from build123d import *

# Parameters (mm, degrees)
SKETCH_1_W          = 20
SKETCH_1_H          = 145
EXTRUDE_1_DEPTH     = 5
SKETCH_3_W          = 20
SKETCH_3_H          = 5
EXTRUDE_2_DEPTH     = 50
SKETCH_4_W          = 20
SKETCH_4_H          = 5
EXTRUDE_3_DEPTH     = 30
SKETCH_5_W          = 20
SKETCH_5_H          = 20
CUT_EXTRUDE_1_DEPTH = 30
SKETCH_6_W          = 20
SKETCH_6_H          = 5
EXTRUDE_4_DEPTH     = 20
SKETCH_7_W          = 20
SKETCH_7_H          = 5
EXTRUDE_5_DEPTH     = 20
EXTRUDE_6_DEPTH     = 2.5
SKETCH_10_R         = 2
CUT_EXTRUDE_2_DEPTH = 5
SKETCH_11_R         = 2
CUT_EXTRUDE_3_DEPTH = 5
SKETCH_12_R         = 2.75
CUT_EXTRUDE_4_DEPTH = 5
SKETCH_13_W         = 20
SKETCH_13_H         = 5
EXTRUDE_7_DEPTH     = 5
SKETCH_14_W         = 20
SKETCH_14_H         = 5
EXTRUDE_8_DEPTH     = 20
SKETCH_15_R         = 2.75
CUT_EXTRUDE_5_DEPTH = 20


with BuildPart() as part:
    # 草图1 → 凸台-拉伸1 (new body)
    with BuildSketch(Plane.XY):
        with Locations((0.170940171, -57.628205128)):
            Rectangle(SKETCH_1_W, SKETCH_1_H)
    extrude(amount=-EXTRUDE_1_DEPTH)

    # 草图3 → 凸台-拉伸2 (add)
    with BuildSketch(Plane(origin=(0, 0, -5), x_dir=(-1, 0, 0), z_dir=(0, 0, -1))):
        with Locations((-0.170940171, 12.371794872)):
            Rectangle(SKETCH_3_W, SKETCH_3_H)
    extrude(amount=EXTRUDE_2_DEPTH)

    # 草图4 → 凸台-拉伸3 (add)
    with BuildSketch(Plane(origin=(0, 0, -5), x_dir=(-1, 0, 0), z_dir=(0, 0, -1))):
        with Locations((-0.170940171, -107.628205128)):
            Rectangle(SKETCH_4_W, SKETCH_4_H)
    extrude(amount=EXTRUDE_3_DEPTH)

    # 草图5 → 切除-拉伸1 (cut)
    with BuildSketch(Plane(origin=(0, 0, -5), x_dir=(-1, 0, 0), z_dir=(0, 0, -1))):
        with Locations((-0.170940171, -120.128205128)):
            Rectangle(SKETCH_5_W, SKETCH_5_H)
    extrude(amount=-CUT_EXTRUDE_1_DEPTH, mode=Mode.SUBTRACT)

    # 草图6 → 凸台-拉伸4 (add)
    with BuildSketch(Plane(origin=(0, -110.128205128, 0), x_dir=(-1, 0, 0), z_dir=(0, -1, 0))):
        with Locations((-0.170940171, 32.5)):
            Rectangle(SKETCH_6_W, SKETCH_6_H)
    extrude(amount=EXTRUDE_4_DEPTH)

    # 草图7 → 凸台-拉伸5 (add)
    with BuildSketch(Plane(origin=(0, 0, -35), x_dir=(-1, 0, 0), z_dir=(0, 0, -1))):
        with Locations((-0.170940171, -127.628205128)):
            Rectangle(SKETCH_7_W, SKETCH_7_H)
    extrude(amount=EXTRUDE_5_DEPTH)

    # 草图9 → 凸台-拉伸6 (add, symmetric)
    with BuildSketch(Plane(origin=(0.170940171, 0, 0), x_dir=(0, 0, -1), z_dir=(1, 0, 0))):
        Polygon((8.965273833, -110.036991646), (29.929169638, -127.991202337), (29.929169638, -110.036991646), align=None)
    extrude(amount=EXTRUDE_6_DEPTH, both=True)

    # 草图10 → 切除-拉伸2 (cut)
    with BuildSketch(Plane.XZ.offset(-9.871794872)):
        with Locations((0.170940171, -17.5)):
            Circle(SKETCH_10_R)
        with Locations((0.170940171, -42.5)):
            Circle(SKETCH_10_R)
    extrude(amount=-CUT_EXTRUDE_2_DEPTH, mode=Mode.SUBTRACT)

    # 草图11 → 切除-拉伸3 (cut)
    with BuildSketch(Plane(origin=(0, 0, -5), x_dir=(-1, 0, 0), z_dir=(0, 0, -1))):
        with Locations((-0.170940171, -22.628205128)):
            Circle(SKETCH_11_R)
        with Locations((-0.170940171, -72.628205128)):
            Circle(SKETCH_11_R)
    extrude(amount=-CUT_EXTRUDE_3_DEPTH, mode=Mode.SUBTRACT)

    # 草图12 → 切除-拉伸4 (cut)
    with BuildSketch(Plane(origin=(0, -125.128205128, 0), x_dir=(1, 0, 0), z_dir=(0, 1, 0))):
        with Locations((0.170940171, 45)):
            Circle(SKETCH_12_R)
    extrude(amount=-CUT_EXTRUDE_4_DEPTH, mode=Mode.SUBTRACT)

    # 草图13 → 凸台-拉伸7 (add)
    with BuildSketch(Plane(origin=(0, 0, -55), x_dir=(-1, 0, 0), z_dir=(0, 0, -1))):
        with Locations((-0.170940171, -127.628205128)):
            Rectangle(SKETCH_13_W, SKETCH_13_H)
    extrude(amount=EXTRUDE_7_DEPTH)

    # 草图14 → 凸台-拉伸8 (add)
    with BuildSketch(Plane(origin=(0, -125.128205128, 0), x_dir=(1, 0, 0), z_dir=(0, 1, 0))):
        with Locations((0.170940171, 57.5)):
            Rectangle(SKETCH_14_W, SKETCH_14_H)
    extrude(amount=EXTRUDE_8_DEPTH)

    # 草图15 → 切除-拉伸5 (cut)
    with BuildSketch(Plane.XY.offset(-55)):
        with Locations((0.170940171, -115.12820513)):
            Circle(SKETCH_15_R)
    extrude(amount=-CUT_EXTRUDE_5_DEPTH, mode=Mode.SUBTRACT)


solid = part.part
Could you check a few things on this model? Use its own coordinates, in mm. A direction names the side the tool comes from. Give positions to 0.01 mm unless a question says otherwise; leave off trailing zeros. Order: outer loops, then holes, each group sorted by start corner. A loop starts at its lowest first (then second) coordinate and runs counter-clockwise, first axis right, second up.
Item 1: If we section it at C-C, the plane x = 7: Write out the boundary of the cut face in (y, z).
Item 2: For faces 4 (the face through (-0.187, -127.593, -47.727)), 5 (the face through (-0.43, -117.81, -57.46)), 6 (the face through (0, -105.128, -58)), 7 (the face through (0, -115, -35)), which set-ups out of +Z, -Z, +X, -X, +Y, -Y let a thin tool reach every point of the face, with its end or its side?
Item 3: I'm going to push flat-ended pins straight in: pin 1 (10 mm diameter, centred on x = -3.5, y = -15, fed in from -Z); pin 2 (3 mm diameter, centred on x = 0.17, z = -42.5, fed in from +Y); pin 3 (1.5 mm diameter, centred on x = 0, y = -117, fed in from -Z). Where does each tip first touch, or does it pass through?
Item 4: If we section it at B-B, the plane z = -17.5: Write out the boundary of the cut face in (x, y), plus the area to 3 significant figures.
Item 5: If we section it at D-D, the plane x = -0.25: Count the separate pieces of the cut face and the enclosed holes in it, plus the area to 3 significant figures.
Item 6: I need wall thicknesses on line 1 (Y direction, x = -2.5, z = -53); line 2 (Y direction, x = 8.75, z = -16.5); line 3 (Z direction, x = -0.5, y = -110). Which ranges of each line are inside material? Lowest first, please.
Item 7: If we section it at A-A, the plane z = -38: Write out the boundary of the cut face in (x, y), plus the area to 3 significant figures.
Item 8: If we mould it in two halves opening along Z, with no side actions, what happens to faces 1 (the face through (2.3, -113, -55)), 2 (the face through (0, -105.128, -20)), 3 (the face through (0, -47, 0))? For each: pulls with the +Z half, pulls with the -Z half, needs draft (parallel to the pull), parting line crosses it, or undercut.
Values:
1. outline: (-130.13, -60) - (-105.13, -60) - (-105.13, -55) - (-125.13, -55) - (-125.13, -35) - (-105.13, -35) - (-105.13, -5) - (9.87, -5) - (9.87, -55) - (14.87, -55) - (14.87, 0) - (-110.13, 0) - (-110.13, -30) - (-130.13, -30) - close
2. face 4: -Y
2. face 5: -Z
2. face 6: -Z, +X, -X, +Y
2. face 7: +X, -X
3. pin 1: stops at z = -5
3. pin 2: stops at y = -125.13
3. pin 3: stops at z = -35
4. outline: (-9.83, -110.13) - (-2.33, -110.13) - (-2.33, -117.35) - (2.67, -117.35) - (2.67, -110.13) - (10.17, -110.13) - (10.17, -105.13) - (-9.83, -105.13) - close; (-9.83, 9.87) - (-1.83, 9.87) - (-1.83, 14.87) - (-9.83, 14.87) - close; (2.17, 9.87) - (10.17, 9.87) - (10.17, 14.87) - (2.17, 14.87) - close
4. area: 216 mm2
5. separate pieces: 7
5. enclosed holes: 0
5. area: 1,400 mm2
6. line 1: y = -130.13 to -125.13, 9.87 to 14.87
6. line 2: y = -110.13 to -105.13, 9.87 to 14.87
6. line 3: z = -60 to -55, -35 to 0
7. outline: (-9.83, -130.13) - (10.17, -130.13) - (10.17, -125.13) - (-9.83, -125.13) - close; (-9.83, 9.87) - (10.17, 9.87) - (10.17, 14.87) - (-9.83, 14.87) - close
7. area: 200 mm2
8. face 1: undercut
8. face 2: needs draft
8. face 3: pulls with the +Z half
